from build123d import *

# Parameters (mm, degrees)
SKETCH1_W           = 36.195
SKETCH1_H           = 5.08
BOSS_EXTRUDE1_DEPTH = 21.59
SKETCH3_W           = 26.035
SKETCH3_H           = 16.51
CUT_EXTRUDE1_DEPTH  = 16.51
SKETCH5_W           = 5.08
SKETCH5_H           = 5.08
BOSS_EXTRUDE2_DEPTH = 5.08
SKETCH6_R           = 1.778
CUT_EXTRUDE2_DEPTH  = 9.144


with BuildPart() as part:
    # Sketch1 → Boss-Extrude1 (new body)
    with BuildSketch(Plane(origin=(0, 0, 0), x_dir=(1, 0, 0), z_dir=(0, 1, 0))):
        with Locations((-4.675909091, -2.54)):
            Rectangle(SKETCH1_W, SKETCH1_H)
    extrude(amount=BOSS_EXTRUDE1_DEPTH)

    # Sketch3 → Cut-Extrude1 (cut)
    with BuildSketch(Plane.XY):
        with Locations((-4.675909091, 8.255)):
            Rectangle(SKETCH3_W, SKETCH3_H)
    extrude(amount=CUT_EXTRUDE1_DEPTH, mode=Mode.SUBTRACT)

    # Sketch5 → Boss-Extrude2 (add)
    with BuildSketch(Plane(origin=(0, 0, 0), x_dir=(1, 0, 0), z_dir=(0, 1, 0))):
        with Locations((-25.313409091, -2.54)):
            Rectangle(SKETCH5_W, SKETCH5_H)
        with Locations((15.961590909, -2.54)):
            Rectangle(SKETCH5_W, SKETCH5_H)
    extrude(amount=BOSS_EXTRUDE2_DEPTH)

    # Sketch6 → Cut-Extrude2 (cut)
    with BuildSketch(Plane(origin=(0, 0, 0), x_dir=(1, 0, 0), z_dir=(0, 1, 0))):
        with Locations(Location((-25.313409091, -2.54, 0), (0, 0, 270))):
            Circle(SKETCH6_R)
        with Locations(Location((15.961590909, -2.54, 0), (0, 0, 90))):
            Circle(SKETCH6_R)
    extrude(amount=CUT_EXTRUDE2_DEPTH, mode=Mode.SUBTRACT)


solid = part.part
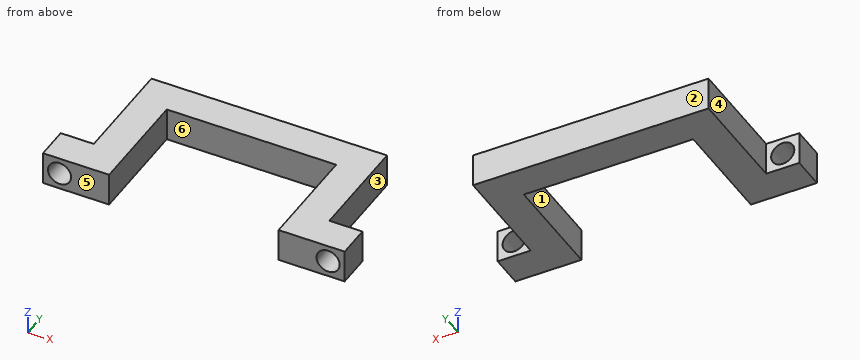
Geometry: final body of the model. Coordinates: model frame, mm. Face numbers are marked on the shaded views. A direction names the side the tool comes from. Round coordinates to 2 decimals unless told otherwise and drop trailing zeros. Loops run counter-clockwise (first coordinate to the right, second up) from the corner with the lowest first, then second, coordinate; pieces in that order, holes last. Notation, with made-up numbers: (71, 45) - (83, 45) arc R15 cw to (83, 66) - close; hole circle Ø9 at (45, -30). An arc over 180 degrees is marked (long way). Write each question's results on one line, items separated by ' | '. Start each with the question number.
1) Access query for the marked faces 4, 5 and 6. Directions: +Z, -Z, +X, -X, +Y, -Y. A direction counts if a zero-diameter tool reaches every point of the face in a straight line with its end or side. Return the directions, or none.
2) Cut plane D-D on x = 16.5. Return loops of the section in (y, z).
3) First-contact query: P1, Ø2, axis at x = -25.31, z = 2.54, coming from the -Y side; P2, Ø2.5, axis at y = 11.5, z = 2.5, coming from the -X side; P3, Ø2.5, axis at x = -8, z = 3, coming from the -Y side; P4, Ø2.5, axis at x = -24.5, z = 2, coming from the +Y side. Flat tips, straight axial feed; report the tip coordinate or a pass-through.
4) Cut plane B-B on y = 11.5. Return loops of the section in (x, z), then the cut area to 3 significant figures.
5) Mould query, pull axis X, two halves, no side actions, for the marked faces 1, 2 and 3. Classes: released by +X, released by -X, zero draft, split by the parting line, or undercut.
6) Cut plane C-C on z = 2.75. Return loops of the section in (x, y), then the cut area to 3 significant figures.
7) Cut plane A-A on y = 1.75. Return loops of the section in (x, z).
8) Line query: probe 1 along X at (y, z) = (8.5, 3.95); probe 2 along X at (y, z) = (3.3, 2.54); probe 3 along X at (y, z) = (1.5, 1.85). Output: solid intervals per line, ascending. Write a range as [from, to].
Verdict:
1) face 4: +Z, -Z, -X, +Y | face 5: +Z, -Z, +X, -X, -Y | face 6: +Z, -Z, -Y
2) outline: (0, 0) - (5.08, 0) - (5.08, 0.85) - (0, 0.85) - close; (0, 4.23) - (5.08, 4.23) - (5.08, 5.08) - (0, 5.08) - close
3) P1: passes through | P2: stops at x = -22.77 | P3: stops at y = 16.51 | P4: stops at y = 5.08
4) outline: (-22.77, 0) - (-17.69, 0) - (-17.69, 5.08) - (-22.77, 5.08) - close; (8.34, 0) - (13.42, 0) - (13.42, 5.08) - (8.34, 5.08) - close | area: 51.6 mm2
5) face 1: undercut | face 2: zero draft | face 3: released by +X
6) outline: (-27.85, 0) - (-27.08, 0) - (-27.08, 5.08) - (-27.85, 5.08) - close; (-23.55, 0) - (-17.69, 0) - (-17.69, 16.51) - (8.34, 16.51) - (8.34, 0) - (14.2, 0) - (14.2, 5.08) - (13.42, 5.08) - (13.42, 21.59) - (-22.77, 21.59) - (-22.77, 5.08) - (-23.55, 5.08) - close; (17.73, 0) - (18.5, 0) - (18.5, 5.08) - (17.73, 5.08) - close | area: 367 mm2
7) outline: (-27.85, 0) - (-17.69, 0) - (-17.69, 5.08) - (-27.85, 5.08) - close; (8.34, 0) - (18.5, 0) - (18.5, 5.08) - (8.34, 5.08) - close; hole circle Ø3.56 at (-25.31, 2.54); hole circle Ø3.56 at (15.96, 2.54)
8) probe 1: x = [-22.77, -17.69], [8.34, 13.42] | probe 2: x = [-27.85, -27.09], [-23.54, -17.69], [8.34, 14.18], [17.74, 18.5] | probe 3: x = [-27.85, -26.95], [-23.67, -17.69], [8.34, 14.32], [17.6, 18.5]
